For this review, take the finished solid that the model builds, in its own axes (mm). A direction names the side the tool comes from. Round coordinates to 2 decimals unless told otherwise and drop trailing zeros. Loops run counter-clockwise (first coordinate to the right, second up) from the corner with the lowest first, then second, coordinate; pieces in that order, holes last.
1) Mouldability with a two-part tool opening along Z and no side actions: class faces 4 (the flat face through (2, 0, -4)), 5 (the flat face through (75, 3, -28)), 6 (the flat face through (-66, 3, 10)) as pulls with the +Z half, pulls with the -Z half, needs draft (parallel to the pull), parting line crosses it, or undercut.
2) Take a section at B-B (z = 50). State the section outline as (x, y) points, then the cut area to 3 significant figures.
3) Take a section at C-C (x = -48). State the section outline as (y, z) points, then the cut area to 3 significant figures.
4) Tool access review of faces 1 (the flat face through (-64, 3, -4.5)), 2 (the flat face through (72, 3, 47)), 3 (the flat face through (16, 3, 66)): name each direction out of +Z, -Z, +X, -X, +Y, -Y from which nothing blocks a thin tool from reaching the whole face with its end or side.
5) Wall thickness on L1, parallel to Z at x = 75, y = 3.95; L2, parallel to X at y = 2.35, z = -3; L3, parallel to X at y = 2.4, z = -75: over which ranges is each line inside the solid? List them lowest first.
6) Take a section at A-A (y = 2.75). Give the number of separate pieces and of enclosed holes in the cut face, then the cut area to 3 significant figures.
7) Insertion check: pin 1 (1.8 mm diameter, centred on y = 2.5, z = 13, fed in from -X); pin 2 (1 mm diameter, centred on x = -17, y = 1.5, fed in from +Z); pin 3 (1.2 mm diameter, centred on y = 1.5, z = 64, fed in from +X); pin 4 (1.5 mm diameter, centred on x = 38.5, z = -35, fed in from -Y). Each pin has a flat end and moves straight along its axis. Give the tip position at first contact, or say it passes through.
```python
from build123d import *

# Parameters (mm, degrees)
SKETCH1_R           = 1.5
BOSS_EXTRUDE1_DEPTH = 6


with BuildPart() as part:
    # Sketch1 → Boss-Extrude1 (new body)
    with BuildSketch(Plane(origin=(0, 0, 0), x_dir=(1, 0, 0), z_dir=(0, 1, 0))):
        Polygon((-72, 72), (-72, 28), (-66, 28), (-66, 4.5), (-62, 4.5), (-62, 6.5), (-59, 6.5), (-59, 4.5), (-56, 4.5), (-56, 1.5), (-59, 1.5), (-59, -0.5), (-62, -0.5), (-62, 1.5), (-66, 1.5), (-66, -22), (-72, -22), (-72, -72), (-22, -72), (-22, -66), (1.5, -66), (1.5, -62), (-0.5, -62), (-0.5, -59), (1.5, -59), (1.5, -56), (4.5, -56), (4.5, -59), (6.5, -59), (6.5, -62), (4.5, -62), (4.5, -66), (28, -66), (28, -72), (72, -72), (72, -22), (78, -22), (78, 28), (72, 28), (72, 72), (28, 72), (28, 78), (-22, 78), (-22, 72), align=None)
        with Locations(Location((3, 75, 0), (0, 0, 270))):
            Circle(SKETCH1_R, mode=Mode.SUBTRACT)
        with Locations(Location((75, 3, 0), (0, 0, 270))):
            Circle(SKETCH1_R, mode=Mode.SUBTRACT)
    extrude(amount=BOSS_EXTRUDE1_DEPTH)


solid = part.part
```
Response:
1. face 4: needs draft
1. face 5: pulls with the -Z half
1. face 6: undercut
2. outline: (-72, 0) - (72, 0) - (72, 6) - (-72, 6) - close
2. area: 864 mm2
3. outline: (0, -72) - (6, -72) - (6, 72) - (0, 72) - close
3. area: 864 mm2
4. face 1: -X, +Y, -Y
4. face 2: +Z, +X, +Y, -Y
4. face 3: +Z, +Y, -Y
5. L1: z = -28 to -4.5, -1.5 to 22
5. L2: x = -56 to 73.5, 76.5 to 78
5. L3: x = -22 to 1.5, 4.5 to 28
6. separate pieces: 1
6. enclosed holes: 2
6. area: 20,600 mm2
7. pin 1: stops at x = -66
7. pin 2: stops at z = 66
7. pin 3: stops at x = 72
7. pin 4: stops at y = 0
